```python
from build123d import *

# Parameters (mm, degrees)
SKETCH1_W           = 66
SKETCH1_H           = 35
BOSS_EXTRUDE1_DEPTH = 5
CUT_EXTRUDE1_DEPTH  = 2.5
SKETCH3_R           = 1.65
CUT_EXTRUDE3_DEPTH  = 75.873226189


with BuildPart() as part:
    # Sketch1 → Boss-Extrude1 (new body)
    with BuildSketch(Plane(origin=(0, 0, 0), x_dir=(1, 0, 0), z_dir=(0, 1, 0))):
        with Locations((33, 17.5)):
            Rectangle(SKETCH1_W, SKETCH1_H)
    extrude(amount=BOSS_EXTRUDE1_DEPTH)

    # Sketch2 → Cut-Extrude1 (cut)
    with BuildSketch(Plane(origin=(0, 5, 0), x_dir=(1, 0, 0), z_dir=(0, 1, 0))):
        Polygon((65.15, 7.017949192), (62.15, 5.285898385), (59.15, 7.017949192), (59.15, 10.482050808), (62.15, 12.214101615), (65.15, 10.482050808), align=None)
        Polygon((3.85, 29.714101615), (0.85, 27.982050808), (0.85, 24.517949192), (3.85, 22.785898385), (6.85, 24.517949192), (6.85, 27.982050808), align=None)
        Polygon((3.85, 5.285898385), (6.85, 7.017949192), (6.85, 10.482050808), (3.85, 12.214101615), (0.85, 10.482050808), (0.85, 7.017949192), align=None)
        Polygon((59.15, 27.982050808), (62.15, 29.714101615), (65.15, 27.982050808), (65.15, 24.517949192), (62.15, 22.785898385), (59.15, 24.517949192), align=None)
    extrude(amount=-CUT_EXTRUDE1_DEPTH, mode=Mode.SUBTRACT)

    # Sketch3 → Cut-Extrude3 (cut, through all)
    with BuildSketch(Plane(origin=(0, 5, 0), x_dir=(1, 0, 0), z_dir=(0, 1, 0))):
        with Locations(Location((3.85, 8.75, 0), (0, 0, 270))):
            Circle(SKETCH3_R)
        with Locations(Location((3.85, 26.25, 0), (0, 0, 270))):
            Circle(SKETCH3_R)
        with Locations(Location((62.15, 26.25, 0), (0, 0, 270))):
            Circle(SKETCH3_R)
        with Locations(Location((62.15, 8.75, 0), (0, 0, 270))):
            Circle(SKETCH3_R)
    extrude(amount=-CUT_EXTRUDE3_DEPTH, mode=Mode.SUBTRACT)


solid = part.part
```
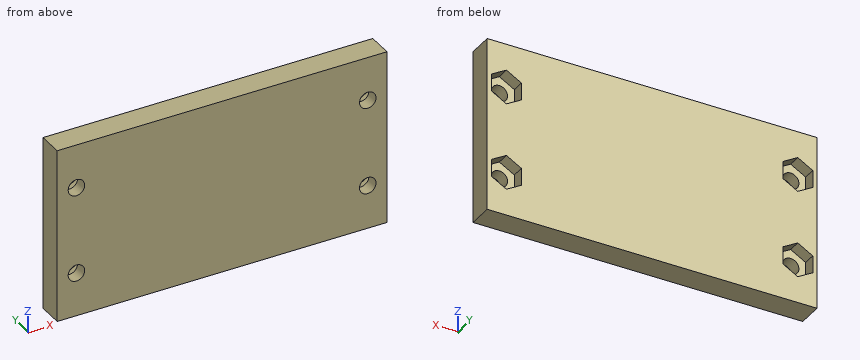
Check sheet for the modelled part. Datum: model origin and axes. Units: mm. Round coordinates to 2 decimals unless told otherwise and drop trailing zeros. Loops run counter-clockwise (first coordinate to the right, second up) from the corner with the lowest first, then second, coordinate; pieces in that order, holes last. Notation, with made-up numbers: (28.25, 43) - (61.25, 43) arc R20 cw to (61.25, 66) - close; hole circle Ø8 at (-26.75, 28). An arc over 180 degrees is marked (long way). Write item = value, one per line. Start each with the question number.
Q1. Section check C-C (z = -27). Record the boundary of the cut face in (x, y).
Q2. Section check B-B (y = 3.6). Record the boundary of the cut face in (x, z).
Q3. Thickness scan on L1, parallel to X at y = 1.25, z = -26.25; L2, parallel to X at y = 3.35, z = -9; L3, parallel to Z at x = 61.5, y = 2.3. Record the ranges inside material, lowest first.
Q4. Section check A-A (z = -8.75). Record the boundary of the cut face in (x, y), plus the area to 4 significant figures.
Q5. Depth check by flat-ended pin: P1, Ø1.2, axis at y = 4, z = -25.5, coming from the -X side; P2, Ø3, axis at x = 63.5, z = -9.5, coming from the +Y side. Enter the tip coordinate at first touch or a pass-through.
Derived:
q1.outline = (0, 0) - (2.38, 0) - (2.38, 2.5) - (0.85, 2.5) - (0.85, 5) - (0, 5) - close; (5.32, 0) - (60.68, 0) - (60.68, 2.5) - (59.15, 2.5) - (59.15, 5) - (6.85, 5) - (6.85, 2.5) - (5.32, 2.5) - close; (63.62, 0) - (66, 0) - (66, 5) - (65.15, 5) - (65.15, 2.5) - (63.62, 2.5) - close
q2.outline = (0, -35) - (66, -35) - (66, 0) - (0, 0) - close; hole (0.85, -27.98) - (3.85, -29.71) - (6.85, -27.98) - (6.85, -24.52) - (3.85, -22.79) - (0.85, -24.52) - close; hole (0.85, -10.48) - (3.85, -12.21) - (6.85, -10.48) - (6.85, -7.02) - (3.85, -5.29) - (0.85, -7.02) - close; hole (59.15, -27.98) - (62.15, -29.71) - (65.15, -27.98) - (65.15, -24.52) - (62.15, -22.79) - (59.15, -24.52) - close; hole (59.15, -10.48) - (62.15, -12.21) - (65.15, -10.48) - (65.15, -7.02) - (62.15, -5.29) - (59.15, -7.02) - close
q3.L1 = 0 to 2.2, 5.5 to 60.5, 63.8 to 66
q3.L2 = 0 to 0.85, 6.85 to 59.15, 65.15 to 66
q3.L3 = -35 to -27.77, -24.73 to -10.27, -7.23 to 0
q4.outline = (0, 0) - (2.2, 0) - (2.2, 2.5) - (0.85, 2.5) - (0.85, 5) - (0, 5) - close; (5.5, 0) - (60.5, 0) - (60.5, 2.5) - (59.15, 2.5) - (59.15, 5) - (6.85, 5) - (6.85, 2.5) - (5.5, 2.5) - close; (63.8, 0) - (66, 0) - (66, 5) - (65.15, 5) - (65.15, 2.5) - (63.8, 2.5) - close
q4.area = 283.5 mm^2
q5.P1 = 0
q5.P2 = 2.5
